```python
from build123d import *

# Parameters (mm, degrees)
SALIENTE_EXTRUIR1_DEPTH = 60


with BuildPart() as part:
    # Croquis1 → Saliente-Extruir1 (new, symmetric)
    with BuildSketch(Plane(origin=(0, 0, 0), x_dir=(0, 0, -1), z_dir=(1, 0, 0))):
        with BuildLine():
            Line((0, 0), (0, 150))
            Line((0, 150), (12.7, 150))
            Line((12.7, 150), (12.7, 22.7))
            ThreePointArc((12.7, 22.7), (15.628932188, 15.628932188), (22.7, 12.7))
            Line((22.7, 12.7), (150, 12.7))
            Line((150, 12.7), (150, 0))
            Line((150, 0), (0, 0))
        make_face()
    extrude(amount=SALIENTE_EXTRUIR1_DEPTH, both=True)


solid = part.part
```
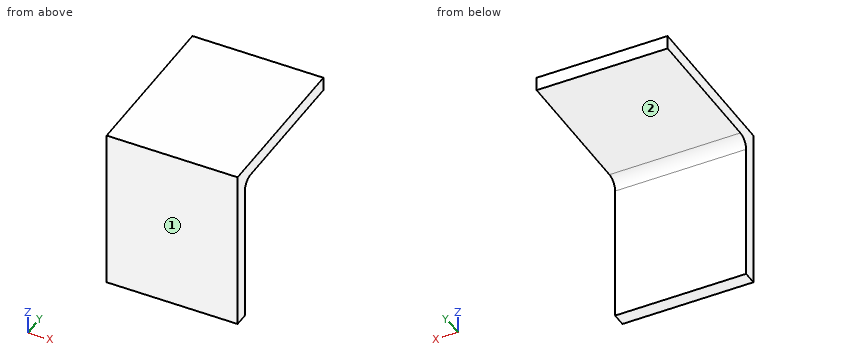
The listing builds one solid part. Answer for the finished solid, in the listing's coordinates (mm). Face numbers are marked on the shaded views. A direction names the side the tool comes from. Give positions to 0.01 mm unless a question says otherwise; leave off trailing zeros. Order: outer loops, then holes, each group sorted by start corner. A loop starts at its lowest first (then second) coordinate and runs counter-clockwise, first axis right, second up.
1) Find section A-A on x = -49.5. Write down the section's boundary in (y, z), then the cut area to 3 significant figures.
Reported:
outline: (0, -150) - (12.7, -150) - (12.7, -22.7) arc R10 cw to (22.7, -12.7) - (150, -12.7) - (150, 0) - (0, 0) - close
area: 3,670 mm2
2) Find section C-C on y = 130.5. Write down the section's boundary in (x, z), then the cut area to 3 significant figures.
Reported:
outline: (-60, -12.7) - (60, -12.7) - (60, 0) - (-60, 0) - close
area: 1,520 mm2
3) For the marked faces 1 and 2, determine the directions among +Z, -Z, +X, -X, +Y, -Y from which every point of the face is accessible in a straight line to the end or side of a thin tool.
Reported:
face 1: +Z, -Z, +X, -X, -Y
face 2: -Z, +X, -X, +Y
4) Find section B-B on z = -127. Write down the section's boundary in (x, y), then the cut area to 3 significant figures.
Reported:
outline: (-60, 0) - (60, 0) - (60, 12.7) - (-60, 12.7) - close
area: 1,520 mm2
5) Given P1, Ø6, axis at x = -12.5, z = -89.5, coming from the +Y side, flat-ended and moving along its own axis, determine where the tip first touches the part or whether it passes through.
Reported:
P1: stops at y = 12.7
6) Consider line 1 along Y through (x, z) = (40, -101.5); line 2 along Z through (x, y) = (-40.5, 141); line 3 along Z through (x, y) = (-36.5, 18). Determine where each line is inside the solid, lowest interval first.
Reported:
line 1: y = 0 to 12.7
line 2: z = -12.7 to 0
line 3: z = -13.87 to 0
